Can you work these out from the model? Positions are in its coordinate system, mm. A direction names the side the tool comes from. Give positions to 0.01 mm unless a question says otherwise; leave off trailing zeros. Order: outer loops, then holes, each group sorted by start corner. A loop starts at its lowest first (then second) coordinate and runs counter-clockwise, first axis right, second up.
Item 1: I want a section at B-B, the plane z = -33.5. Write out the boundary of the cut face in (x, y).
Item 2: I'm going to push flat-ended pins straight in: pin 1 Ø0.5 at (y, z) = (-44.5, -38) entering from +X; pin 2 Ø4 at (x, y) = (0.5, -35.5) entering from +Z; pin 3 Ø4 at (x, z) = (0, 33.5) entering from +Y; pin 4 Ø2 at (x, y) = (1, -22.5) entering from -Z. Where does each tip first touch, or does it pass through?
Item 3: I want a section at D-D, the plane z = 6.5. Write out the boundary of the cut face in (x, y).
Item 4: I want a section at A-A, the plane x = 0. Count the separate pieces of the cut face and the enclosed holes in it, then the cut area to 3 significant figures.
Item 5: If we mould it in two halves opening along Z, with no side actions, what happens to faces 4 (the flat face through (-2.75, -3.45, 20.75)), 5 (the flat face through (0, -27, -28)), 6 (the flat face through (-2.75, -44.31, 25.16))? For each: +Z half, -Z half, draft (parallel to the pull), parting line (faces both ways), or undercut.
Item 6: I want a section at C-C, the plane y = -40. Write out the boundary of the cut face in (x, z).
Item 7: Which directions (+Z, -Z, +X, -X, +Y, -Y) give clear straight access to the entire face, cutting with the end or side of a thin tool? Please do faces 1 (the flat face through (3, -43.5, 33)), 2 (the flat face through (-2.75, -5.74, -18.09)), 3 (the flat face through (0, -44.5, -25)).
Item 8: If I drill on line 1 along X through (y, z) = (-44.85, -33.5); line 2 along Z through (x, y) = (-0.25, -41); line 3 along X through (y, z) = (1, -3.5), over which ranges is the centre line in solid material (lowest first)?
```python
from build123d import *

# Parameters (mm, degrees)
SKETCH1_W           = 6
SKETCH1_H           = 24
SKETCH1_R           = 1.55
BOSS_EXTRUDE1_DEPTH = 4
BOSS_EXTRUDE2_DEPTH = 6
SKETCH3_R           = 2.25
CUT_EXTRUDE1_DEPTH  = 62.532511732
BOSS_EXTRUDE3_DEPTH = 2
CHAMFER1_SIZE       = 0.5


with BuildPart() as part:
    # Sketch1 → Boss-Extrude1 (new body)
    with BuildSketch(Plane(origin=(0, 0, 0), x_dir=(1, 0, 0), z_dir=(0, 1, 0))):
        Rectangle(SKETCH1_W, SKETCH1_H)
        with Locations(Location((0, 0, 0), (0, 0, 270))):
            Circle(SKETCH1_R, mode=Mode.SUBTRACT)
    extrude(amount=BOSS_EXTRUDE1_DEPTH)

    # Sketch2 → Boss-Extrude2 (add)
    with BuildSketch(Plane.ZY.offset(3)):
        Polygon((-12, 0), (-24, -12), (-24, -43.5), (-26, -45.5), (-39, -45.5), (-39, -43.5), (-28, -43.5), (-28, -10.343145751), (-13.656854249, 4), (-12, 4), align=None)
    boss_extrude2 = extrude(amount=-BOSS_EXTRUDE2_DEPTH)

    # Sketch3 → Cut-Extrude1 (cut, through all)
    with BuildSketch(Plane(origin=(0, -43.5, 0), x_dir=(1, 0, 0), z_dir=(0, 1, 0))):
        with Locations(Location((0, 33.5, 0), (0, 0, 270))):
            Circle(SKETCH3_R)
    cut_extrude1 = extrude(amount=-CUT_EXTRUDE1_DEPTH, mode=Mode.SUBTRACT)

    # Sketch4 → Boss-Extrude3 (add)
    with BuildSketch(Plane(origin=(0, -43.5, 0), x_dir=(1, 0, 0), z_dir=(0, 1, 0))):
        with BuildLine():
            Line((3, 29.5), (3, 37.5))
            ThreePointArc((3, 37.5), (5, 33.5), (3, 29.5))
        make_face()
    boss_extrude3 = extrude(amount=-BOSS_EXTRUDE3_DEPTH)

    # Mirror1: Boss-Extrude2, Cut-Extrude1, Boss-Extrude3 across plane
    add(boss_extrude2.mirror(Plane.XY))
    add(cut_extrude1.mirror(Plane.XY), mode=Mode.SUBTRACT)
    add(boss_extrude3.mirror(Plane.XY))

    # Chamfer1
    chamfer1_edges = [part.edges().sort_by_distance(p)[0] for p in [
        (-3, 4, 0),
        (0, -45.5, -39),
        (0, -43.5, -39),
        (-3, -3.171572875, -20.828427125),
        (-3, -26.921572875, -28),
        (-3, -43.5, -33.5),
        (-3, -44.5, -39),
        (-3, -45.5, -32.5),
        (-3, -44.5, -25),
        (-3, -27.75, -24),
        (-3, -6, -18),
        (3, -6, -18),
        (3, -27.75, -24),
        (3, -44.5, -25),
        (3, -45.5, -27.75),
        (3, -44.5, -39),
        (3, -43.5, -38.25),
        (3, -26.921572875, -28),
        (3, -3.171572875, -20.828427125),
        (3, -43.5, -28.75),
        (3, -45.5, -38.25),
        (5, -43.5, -33.5),
        (5, -45.5, -33.5),
        (3, 4, 0),
        (-3, 0, 0),
        (3, -6, 18),
        (-3, -6, 18),
        (3, -27.75, 24),
        (-3, -27.75, 24),
        (3, -44.5, 25),
        (-3, -44.5, 25),
        (3, -45.5, 27.75),
        (0, -45.5, 39),
        (-3, -45.5, 32.5),
        (3, -44.5, 39),
        (0, -43.5, 39),
        (-3, -44.5, 39),
        (3, -43.5, 38.25),
        (-3, -43.5, 33.5),
        (3, -26.921572875, 28),
        (-3, -26.921572875, 28),
        (3, -3.171572875, 20.828427125),
        (-3, -3.171572875, 20.828427125),
        (3, 0, 0),
        (3, -43.5, 28.75),
        (3, -45.5, 38.25),
        (5, -43.5, 33.5),
        (5, -45.5, 33.5),
    ]]
    chamfer(chamfer1_edges, length=CHAMFER1_SIZE)


solid = part.part
```
Results list:
1. outline: (-3, -45) - (-2.5, -45.5) - (-2.25, -45.5) - (-2.25, -43.5) - (-2.5, -43.5) - (-3, -44) - close; (2.25, -45.5) - (4.5, -45.5) - (5, -45) - (5, -44) - (4.5, -43.5) - (2.25, -43.5) - close
2. pin 1: stops at x = 3
2. pin 2: stops at z = 28
2. pin 3: passes through
2. pin 4: stops at z = -28
3. outline: (-3, 0.5) - (-2.5, 0) - (2.5, 0) - (3, 0.5) - (3, 3.5) - (2.5, 4) - (-2.5, 4) - (-3, 3.5) - close
4. separate pieces: 4
4. enclosed holes: 0
4. area: 535 mm2
5. face 4: +Z half
5. face 5: -Z half
5. face 6: undercut
6. outline: (-3, -27.5) - (-2.5, -28) - (2.5, -28) - (3, -27.5) - (3, -24.5) - (2.5, -24) - (-2.5, -24) - (-3, -24.5) - close; (-3, 24.5) - (-2.5, 24) - (2.5, 24) - (3, 24.5) - (3, 27.5) - (2.5, 28) - (-2.5, 28) - (-3, 27.5) - close
7. face 1: +Z, +X, -X, +Y
7. face 2: -X, -Y
7. face 3: +X, -X, -Y
8. line 1: x = -3 to -2.25, 2.25 to 5
8. line 2: z = -28 to -24, 24 to 28
8. line 3: x = -3 to 3
